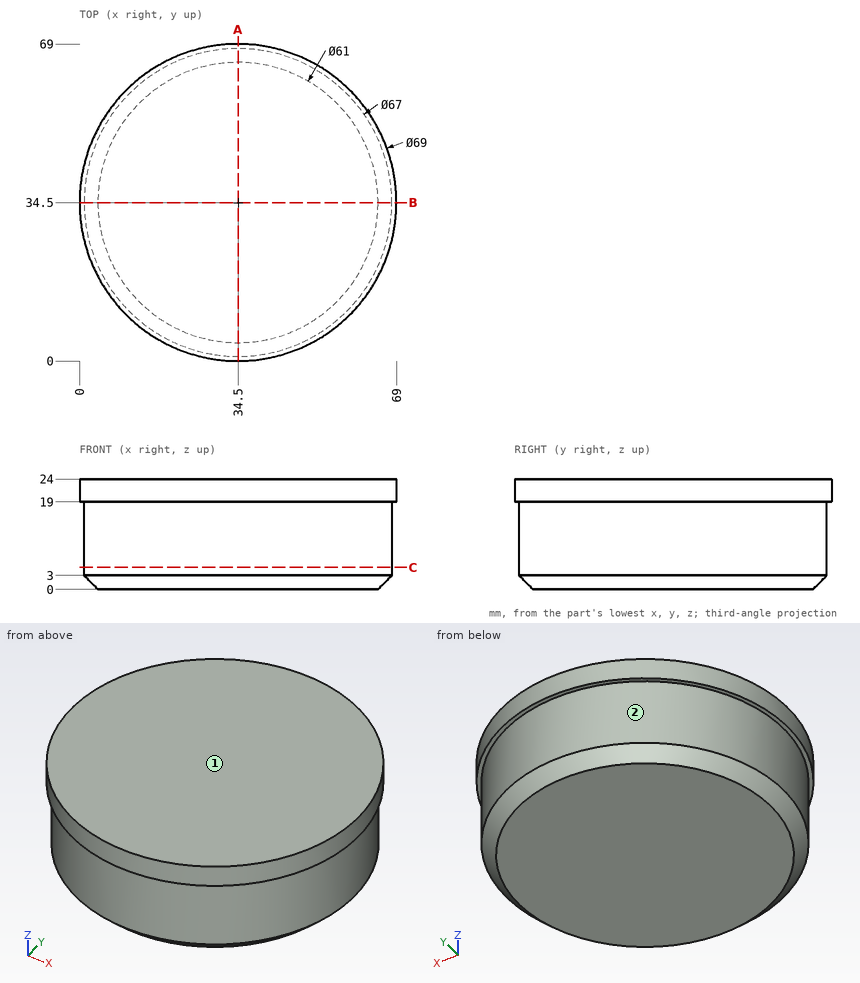
Geometry check sheet. Reference: drawing and pictorial views, mm from the part's lowest x, y, z. A direction names the side the tool comes from. Give positions to 0.01 mm unless a question says otherwise; leave off trailing zeros. Order: outer loops, then holes, each group sorted by start corner. A loop starts at its lowest first (then second) coordinate and runs counter-clockwise, first axis right, second up. Notation, with made-up numbers: (-29, 21) - (17, 21) arc R12 ccw to (17, 37) - close; hole circle Ø6 at (89, -5). An arc over 180 degrees is marked (long way). Answer as CSV lines item,"result". Start each with the question number.
Item 1: Material ranges on L1, parallel to Y at x = 36, z = 8.5; L2, parallel to X at y = 17, z = 22; L3, parallel to Y at x = 50.5, z = 21.5, recorded low to high.
Item 2: Access from +Z, -Z, +X, -X, +Y, -Y to the whole of each face (thin tool, end or side, straight path). Record for the marked faces 1 and 2.
Item 3: Gauge pin test, flat ends, axial feed: pin 1 (6 mm diameter, centred on y = 48, z = 3, fed in from +X); pin 2 (8 mm diameter, centred on x = 29, z = 3.5, fed in from -Y); pin 3 (2 mm diameter, centred on x = 10.5, z = 6, fed in from +Y). Record the tip position at first contact, or that the pin passes through.
Item 4: Section check A-A, the plane x = 34.5. Record the boundary of the cut face in (y, z), plus the area to 3 significant figures.
Item 5: Section check C-C, the plane z = 4.75. Record the boundary of the cut face in (x, y).
Filled in:
1,L1,"1.03 to 67.97"
1,L2,"4.77 to 64.23"
1,L3,"3.93 to 65.07"
2,face 1,"+Z, +X, -X, +Y, -Y"
2,face 2,"-Z"
3,pin 1,"x = 66.31"
3,pin 2,"y = 1.03"
3,pin 3,"y = 58.86"
4,outline,"(0, 19) - (1, 19) - (1, 3) - (4, 0) - (65, 0) - (68, 3) - (68, 19) - (69, 19) - (69, 24) - (0, 24) - close"
4,area,"1,610 mm^2"
5,outline,"circle Ø67 at (34.5, 34.5)"
